The model under review builds one solid part; all positions refer to its coordinate system, in mm. Face numbers are marked on the shaded views. A direction names the side the tool comes from. Coordinates: 2 decimals unless noted, no trailing zeros. Loops run counter-clockwise (first coordinate to the right, second up) from the corner with the lowest first, then second, coordinate; pieces in that order, holes last. Notation, with made-up numbers: M 26,-39 L 53,-39 A27 cw 53,-1 Z; hole C 75.25,38.25 d11. An arc over 180 degrees is marked long. Write item = value, one per line. Start each with the question number.
Q1. For the marked faces 4, 5, 6 and 7, list the 3-axis set-ups (+Z, -Z, +X, -X, +Y, -Y) from which the entire face can be reached by the end or side of a thin tool; tool diameter is ignored.
Q2. We need section D-D on y = -57. Give the boundary of the cut face in (x, z).
Q3. Clearance check with flat-ended pins moving along their axes: pin 1 Ø20.5 at (x, y) = (-11.5, -49) entering from +Z; pin 2 Ø12.5 at (x, z) = (-88, 17) entering from +Y; pin 3 Ø6 at (x, y) = (-16, -67) entering from -Z. State where each tip first meets the part, or that it passes through.
Q4. Wall thickness on probe 1 along Y at (x, z) = (-9, 89.5); probe 2 along X at (y, z) = (-4.5, 23.5); probe 3 along X at (y, z) = (-6, 38): over which ranges is each line inside the solid? List them lowest first.
Q5. Mouldability with a two-part tool opening along Y and no side actions: class the marked faces 1, 2 and 3 as released by +Y, released by -Y, zero draft, split by the parting line, or undercut.
Q6. We need section A-A on z = 85.5. Give the boundary of the cut face in (x, y), and give its area (3 significant figures).
Q7. We need section C-C on z = 30. Give the boundary of the cut face in (x, y), and give its area (3 significant figures).
Q8. We need section B-B on y = -18.5. Give the boundary of the cut face in (x, z).
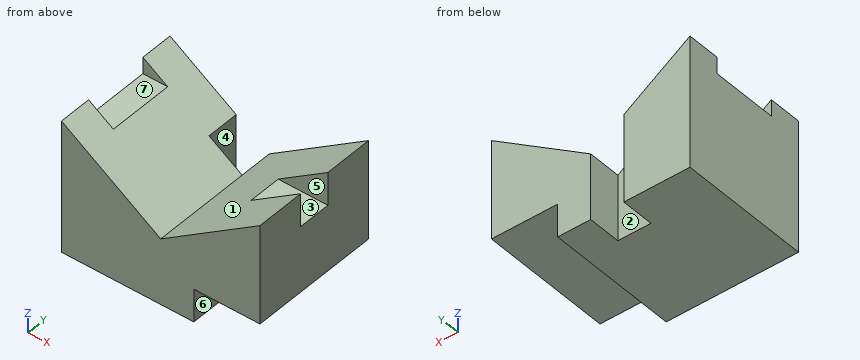
from build123d import *

# Parameters (mm, degrees)
F1_DEPTH = 101.6
F2_W     = 25.4
F2_H     = 25.4
F2_W_2   = 101.6
F3_DEPTH = 50.8
F4_W     = 25.4
F4_H     = 25.4
F5_DEPTH = 101.601
F6_W     = 50.8
F6_H     = 12.7
F7_DEPTH = 25.4


with BuildPart() as f1:
    # F0 (on Front) → F1 (new body)
    with BuildSketch(Plane.XZ):
        Polygon((-152.4, 0), (0, 0), (-76.2, 50.8), align=None)
        Polygon((-76.2, 50.8), (0, 0), (0, 101.6), align=None)
        Polygon((-152.4, 101.6), (-152.4, 0), (-76.2, 50.8), align=None)
    extrude(amount=F1_DEPTH)

    # F2 (on face) → F3 (cut)
    with BuildSketch(Plane.YZ):
        with Locations((-50.8, 88.9)):
            Rectangle(F2_W, F2_H)
        with Locations((-50.8, 12.7)):
            Rectangle(F2_W_2, F2_H)
    extrude(amount=-F3_DEPTH, mode=Mode.SUBTRACT)

    # F4 (on face) → F5 (cut, through all)
    with BuildSketch(Plane(origin=(0, 0, 0), x_dir=(1, 0, 0), z_dir=(0, 0, -1))):
        with Locations((-88.9, 12.7)):
            Rectangle(F4_W, F4_H)
    extrude(amount=-F5_DEPTH, mode=Mode.SUBTRACT)

    # F6 (on face) → F7 (cut)
    with BuildSketch(Plane(origin=(-152.4, 0, 0), x_dir=(0, -1, 0), z_dir=(-1, 0, 0))):
        with Locations((50.8, 95.25)):
            Rectangle(F6_W, F6_H)
    extrude(amount=-F7_DEPTH, mode=Mode.SUBTRACT)


solid = f1.part
Returned:
q1.face_4 = +Z, -Z, +Y
q1.face_5 = +Z, +X
q1.face_6 = -Z, +X, +Y, -Y
q1.face_7 = +Z, -X
q2.outline = M -152.4,0 L -50.8,0 L -50.8,25.4 L 0,25.4 L 0,76.2 L -38.1,76.2 L -76.2,50.8 L -133.35,88.9 L -152.4,88.9 Z
q3.pin_1 = 76.2
q3.pin_2 = -25.4
q3.pin_3 = 25.4
q4.probe_1 = -101.6 to -63.5, -38.1 to 0
q4.probe_2 = -152.4 to -101.6, -76.2 to -50.8
q4.probe_3 = -152.4 to -101.6, -76.2 to 0
q5.face_1 = zero draft
q5.face_2 = released by +Y
q5.face_3 = undercut
q6.outline = M -152.4,-101.6 L -128.25,-101.6 L -128.25,0 L -152.4,0 Z; M -24.15,-101.6 L 0,-101.6 L 0,-63.5 L -24.15,-63.5 Z; M -24.15,-38.1 L 0,-38.1 L 0,0 L -24.15,0 Z
q6.area = 4,290 mm^2
q7.outline = M -152.4,-101.6 L 0,-101.6 L 0,0 L -76.2,0 L -76.2,-25.4 L -101.6,-25.4 L -101.6,0 L -152.4,0 Z
q7.area = 14,800 mm^2
q8.outline = M -152.4,0 L -101.6,0 L -101.6,67.73 L -152.4,101.6 Z; M -76.2,0 L -50.8,0 L -50.8,25.4 L 0,25.4 L 0,101.6 L -76.2,50.8 Z
